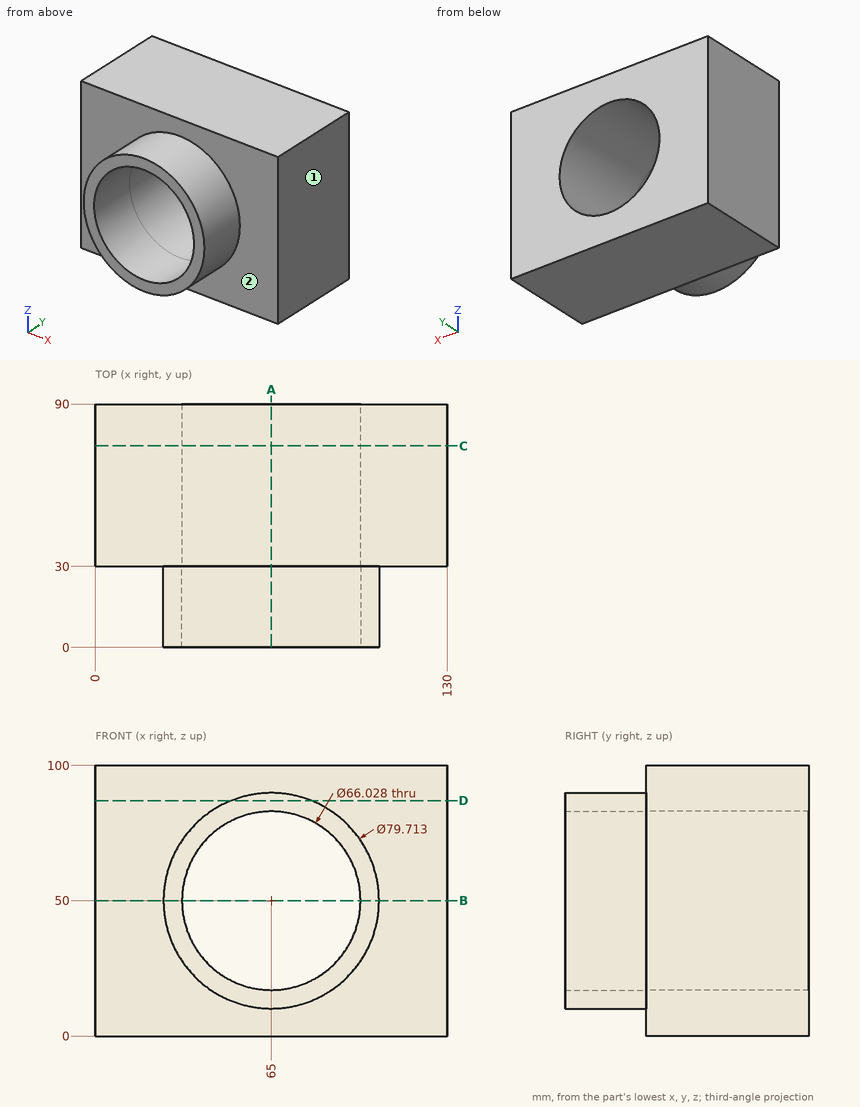
Part print with two shaded views. Sizes in mm from the minimum x, y, z corner. A direction names the side the tool comes from. Coordinates: 2 decimals unless noted, no trailing zeros. Order: outer loops, then holes, each group sorted by start corner. A loop starts at its lowest first (then second) coordinate and runs counter-clockwise, first axis right, second up. Notation, with made-up numbers: M -28.75,84.25 L 2.25,84.25 A28 cw 2.25,104.25 Z; hole C 13.5,-7.75 d6. An arc over 180 degrees is marked long. One line per question, with ' | ' between items. Start each with the question number.
1. Cut at B-B (z = 50). Write the cut outline in (x, y), plus the area to 3 significant figures.
2. Cut at D-D (z = 87). Write the cut outline in (x, y), plus the area to 3 significant figures.
3. Cut at A-A (x = 65). Write the cut outline in (y, z).
4. Tool access for the marked faces 1 and 2: list every direction of +Z, -Z, +X, -X, +Y, -Y with a clear straight run to the whole face (end or side of a thin tool).
5. Flat gauge pins, fed straight in: P1, Ø6, axis at y = 55.5, z = 30.5, coming from the -X side; P2, Ø1, axis at x = 98, y = 18.5, coming from the -Z side; P3, Ø4, axis at y = 26.5, z = 86, coming from the -X side; P4, Ø5, axis at y = 14.5, z = 14, coming from the -X side (1 decimal). Where does each tip first touch, or does it go through?
6. Cut at C-C (y = 74.5). Write the cut outline in (x, z), plus the area to 3 significant figures.
7. Wall check: line 1 along X through (y, z) = (52, 51.5); line 2 along Z through (x, y) = (65, 13); line 3 along Z through (x, y) = (65, 63). Give the ranges that are in metal, low to high. Write a range as [from, to].
The answers:
1) outline: M 0,30 L 25.14,30 L 25.14,0 L 31.99,0 L 31.99,90 L 0,90 Z; M 98.01,0 L 104.86,0 L 104.86,30 L 130,30 L 130,90 L 98.01,90 Z | area: 4,250 mm2
2) outline: M 0,30 L 50.18,30 L 50.18,0 L 79.82,0 L 79.82,30 L 130,30 L 130,90 L 0,90 Z | area: 8,690 mm2
3) outline: M 0,10.14 L 30,10.14 L 30,0 L 90,0 L 90,16.99 L 0,16.99 Z; M 0,83.01 L 90,83.01 L 90,100 L 30,100 L 30,89.86 L 0,89.86 Z
4) face 1: +Z, -Z, +X, +Y, -Y | face 2: -Y
5) P1: stops at x = 0 | P2: stops at z = 26.93 | P3: stops at x = 44.2 | P4: stops at x = 43.4
6) outline: M 0,0 L 130,0 L 130,100 L 0,100 Z; hole C 65,50 d66.03 | area: 9,580 mm2
7) line 1: x = [0, 32.02], [97.98, 130] | line 2: z = [10.14, 16.99], [83.01, 89.86] | line 3: z = [0, 16.99], [83.01, 100]
